```python
from build123d import *

# Parameters (mm, degrees)
SKETCH_1_R          = 135
EXTRUDE_1_DEPTH     = 2
SKETCH_562_R        = 1.6
SKETCH_562_W        = 21
SKETCH_562_H        = 44
CUT_EXTRUDE_1_DEPTH = 10
SKETCH_1031_R       = 1.6
CUT_EXTRUDE_2_DEPTH = 10
SKETCH_4_R          = 2
SKETCH_4_R_2        = 3
SKETCH_4_R_3        = 1.6
CUT_EXTRUDE_3_DEPTH = 10
CUT_EXTRUDE_4_DEPTH = 10
SKETCH_6_R          = 1.6
CUT_EXTRUDE_7_DEPTH = 10


with BuildPart() as part:
    # 草图1 → 凸台-拉伸1 (new body)
    with BuildSketch(Plane(origin=(0, 0, 0), x_dir=(1, 0, 0), z_dir=(0, 1, 0))):
        with Locations(Location((0, 0, 0), (0, 0, 270))):
            Circle(SKETCH_1_R)
    extrude(amount=EXTRUDE_1_DEPTH)

    # Sketch 562 → 切除-拉伸1 (cut)
    with BuildSketch(Plane(origin=(0, 2, 0), x_dir=(1, 0, 0), z_dir=(0, 1, 0))):
        with Locations(Location((-5, 64.75, 0), (0, 0, 270))):
            Circle(SKETCH_562_R)
        with Locations(Location((5, 64.75, 0), (0, 0, 270))):
            Circle(SKETCH_562_R)
        with Locations(Location((-5, 15.25, 0), (0, 0, 270))):
            Circle(SKETCH_562_R)
        with Locations(Location((5, 15.25, 0), (0, 0, 270))):
            Circle(SKETCH_562_R)
        with Locations(Location((18.5, 48.5, 0), (0, 0, 270))):
            Circle(SKETCH_562_R)
        with Locations(Location((18.5, 11.5, 0), (0, 0, 270))):
            Circle(SKETCH_562_R)
        with Locations(Location((-18.5, 11.5, 0), (0, 0, 270))):
            Circle(SKETCH_562_R)
        with Locations(Location((-18.5, 48.5, 0), (0, 0, 270))):
            Circle(SKETCH_562_R)
        with Locations((0, 40)):
            Rectangle(SKETCH_562_W, SKETCH_562_H)
    extrude(amount=-CUT_EXTRUDE_1_DEPTH, mode=Mode.SUBTRACT)

    # Sketch 1031 → 切除-拉伸2 (cut)
    with BuildSketch(Plane(origin=(0, 2, 0), x_dir=(1, 0, 0), z_dir=(0, 1, 0))):
        with Locations(Location((-60, -25, 0), (0, 0, 270))):
            Circle(SKETCH_1031_R)
        with Locations(Location((-40, -25, 0), (0, 0, 270))):
            Circle(SKETCH_1031_R)
        with Locations(Location((40, -25, 0), (0, 0, 270))):
            Circle(SKETCH_1031_R)
        with Locations(Location((60, -25, 0), (0, 0, 270))):
            Circle(SKETCH_1031_R)
        with Locations(Location((60, -105, 0), (0, 0, 270))):
            Circle(SKETCH_1031_R)
        with Locations(Location((40, -105, 0), (0, 0, 270))):
            Circle(SKETCH_1031_R)
        with Locations(Location((-40, -105, 0), (0, 0, 270))):
            Circle(SKETCH_1031_R)
        with Locations(Location((-60, -105, 0), (0, 0, 270))):
            Circle(SKETCH_1031_R)
        with Locations(Location((-42.5, -89.5, 0), (0, 0, 270))):
            Circle(SKETCH_1031_R)
        with Locations(Location((-42.5, -40.5, 0), (0, 0, 270))):
            Circle(SKETCH_1031_R)
        with Locations(Location((15.5, -40.5, 0), (0, 0, 270))):
            Circle(SKETCH_1031_R)
        with Locations(Location((15.5, -89.5, 0), (0, 0, 270))):
            Circle(SKETCH_1031_R)
    extrude(amount=-CUT_EXTRUDE_2_DEPTH, mode=Mode.SUBTRACT)

    # 草图4 → 切除-拉伸3 (cut)
    with BuildSketch(Plane(origin=(0, 2, 0), x_dir=(1, 0, 0), z_dir=(0, 1, 0))):
        with Locations(Location((-72, 97, 0), (0, 0, 270))):
            Circle(SKETCH_4_R)
        with Locations(Location((72, 97, 0), (0, 0, 270))):
            Circle(SKETCH_4_R)
        with Locations(Location((72, -97, 0), (0, 0, 270))):
            Circle(SKETCH_4_R)
        with Locations(Location((-72, -97, 0), (0, 0, 270))):
            Circle(SKETCH_4_R)
        with Locations(Location((0, -120, 0), (0, 0, 270))):
            Circle(SKETCH_4_R_2)
        with Locations(Location((-5.656854249, -125.656854249, 0), (0, 0, 270))):
            Circle(SKETCH_4_R_3)
        with Locations(Location((-5.656854249, -114.343145751, 0), (0, 0, 270))):
            Circle(SKETCH_4_R_3)
        with Locations(Location((5.656854249, -114.343145751, 0), (0, 0, 270))):
            Circle(SKETCH_4_R_3)
        with Locations(Location((5.656854249, -125.656854249, 0), (0, 0, 270))):
            Circle(SKETCH_4_R_3)
        with Locations(Location((5.656854249, 125.656854249, 0), (0, 0, 270))):
            Circle(SKETCH_4_R_3)
        with Locations(Location((5.656854249, 114.343145751, 0), (0, 0, 270))):
            Circle(SKETCH_4_R_3)
        with Locations(Location((-5.656854249, 114.343145751, 0), (0, 0, 270))):
            Circle(SKETCH_4_R_3)
        with Locations(Location((-5.656854249, 125.656854249, 0), (0, 0, 270))):
            Circle(SKETCH_4_R_3)
        with Locations(Location((0, 120, 0), (0, 0, 270))):
            Circle(SKETCH_4_R_2)
        with BuildLine():
            Line((-20, -12.5), (20, -12.5))
            ThreePointArc((20, -12.5), (27.5, -20), (20, -27.5))
            Line((20, -27.5), (-20, -27.5))
            ThreePointArc((-20, -27.5), (-27.5, -20), (-20, -12.5))
        make_face()
    extrude(amount=-CUT_EXTRUDE_3_DEPTH, mode=Mode.SUBTRACT)

    # 草图5 → 切除-拉伸4 (cut)
    with BuildSketch(Plane(origin=(0, 2, 0), x_dir=(1, 0, 0), z_dir=(0, 1, 0))):
        with BuildLine():
            Line((-31.36862915, 63.63137085), (-17.36862915, 49.63137085))
            ThreePointArc((-17.36862915, 49.63137085), (-17.36862915, 47.36862915), (-19.63137085, 47.36862915))
            Line((-19.63137085, 47.36862915), (-33.63137085, 61.36862915))
            ThreePointArc((-33.63137085, 61.36862915), (-33.63137085, 63.63137085), (-31.36862915, 63.63137085))
        make_face()
        with BuildLine():
            Line((33.63137085, 61.36862915), (19.63137085, 47.36862915))
            ThreePointArc((19.63137085, 47.36862915), (17.36862915, 47.36862915), (17.36862915, 49.63137085))
            Line((17.36862915, 49.63137085), (31.36862915, 63.63137085))
            ThreePointArc((31.36862915, 63.63137085), (33.63137085, 63.63137085), (33.63137085, 61.36862915))
        make_face()
        with BuildLine():
            Line((31.36862915, -3.63137085), (17.36862915, 10.36862915))
            ThreePointArc((17.36862915, 10.36862915), (17.36862915, 12.63137085), (19.63137085, 12.63137085))
            Line((19.63137085, 12.63137085), (33.63137085, -1.36862915))
            ThreePointArc((33.63137085, -1.36862915), (33.63137085, -3.63137085), (31.36862915, -3.63137085))
        make_face()
        with BuildLine():
            Line((-33.63137085, -1.36862915), (-19.63137085, 12.63137085))
            ThreePointArc((-19.63137085, 12.63137085), (-17.36862915, 12.63137085), (-17.36862915, 10.36862915))
            Line((-17.36862915, 10.36862915), (-31.36862915, -3.63137085))
            ThreePointArc((-31.36862915, -3.63137085), (-33.63137085, -3.63137085), (-33.63137085, -1.36862915))
        make_face()
    extrude(amount=-CUT_EXTRUDE_4_DEPTH, mode=Mode.SUBTRACT)

    # 草图6 → 切除-拉伸7 (cut)
    with BuildSketch(Plane(origin=(0, 2, 0), x_dir=(1, 0, 0), z_dir=(0, 1, 0))):
        with Locations(Location((71.537199543, 2.5, 0), (0, 0, 270))):
            Circle(SKETCH_6_R)
        with Locations(Location((90.537199543, 2.5, 0), (0, 0, 270))):
            Circle(SKETCH_6_R)
        with Locations(Location((90.537199543, 57.5, 0), (0, 0, 270))):
            Circle(SKETCH_6_R)
        with Locations(Location((71.537199543, 57.5, 0), (0, 0, 270))):
            Circle(SKETCH_6_R)
        with Locations(Location((-95.215957975, -4.25, 0), (0, 0, 270))):
            Circle(SKETCH_6_R)
        with Locations(Location((-56.715957975, -4.25, 0), (0, 0, 270))):
            Circle(SKETCH_6_R)
        with Locations(Location((-95.215957975, 64.25, 0), (0, 0, 270))):
            Circle(SKETCH_6_R)
        with Locations(Location((-56.715957975, 64.25, 0), (0, 0, 270))):
            Circle(SKETCH_6_R)
        with BuildLine():
            add(Edge.make_bspline(
                [(-58.031053316, 15), (-47.63874847, 15), (-52.834900893, 37.5), (-58.031053316, 60), (-63.227205738, 37.5), (-68.423358161, 15), (-58.031053316, 15)],
                knots=[0, 0, 0, 2.094395102, 2.094395102, 4.188790205, 4.188790205, 6.283185307, 6.283185307, 6.283185307], degree=2, weights=[1, 0.5, 1, 0.5, 1, 0.5, 1]))
        make_face()
        with BuildLine():
            add(Edge.make_bspline(
                [(58.031053316, 45), (47.63874847, 45), (52.834900893, 22.5), (58.031053316, 0), (63.227205738, 22.5), (68.423358161, 45), (58.031053316, 45)],
                knots=[0, 0, 0, 2.094395102, 2.094395102, 4.188790205, 4.188790205, 6.283185307, 6.283185307, 6.283185307], degree=2, weights=[1, 0.5, 1, 0.5, 1, 0.5, 1]))
        make_face()
    extrude(amount=-CUT_EXTRUDE_7_DEPTH, mode=Mode.SUBTRACT)


solid = part.part
```
Work out the finished part from the listing and answer in its coordinate system (mm). A direction names the side the tool comes from. Give positions to 0.01 mm unless a question says otherwise; leave off trailing zeros. Loops run counter-clockwise (first coordinate to the right, second up) from the corner with the lowest first, then second, coordinate; pieces in that order, holes last. Notation, with made-up numbers: (-16, -26) -> (35, -26) arc R21 cw to (35, 3) -> close; hole circle Ø2 at (-38, 19.25). An arc over 180 degrees is marked (long way). Put each result on its own line as item: value. Start each with the question number.
Item 1: This flat-tipped pin is pushed along its axis until it touches: P1, Ø1, axis at y = 1, z = -11, coming from the -X side. Where does it stop, or does it pass through?
Item 2: Which of the six approach directions +Z, -Z, +X, -X, +Y, -Y give full straight-line access (tool end or side, diameter ignored) to faces 1 (the face through (2, 0, -2)), 2 (the face through (24.27, 1.01, -56.53))?
Item 3: Find the intervals of material crossed by L1, parallel to X at y = 0.5, z = 25 (3 decimals); L2, parallel to Z at x = 91, y = 1.6; L3, parallel to X at y = 1.45, z = -57.5, in increasing order. Write a range as [from, to].
Item 4: The mould has two halves that part along X. Classify faces 3 (the face through (-119.77, 0.99, 62.29)), 4 (the face through (-24.47, 1.01, -56.73)), 5 (the face through (2, 2, -2)): released by +X, released by -X, zero draft, split by the parting line, or undercut.
Item 5: The part is cut by section A-A (x = -108). Give the vertices of the cut face in (y, z).
Item 6: The part is cut by section D-D (z = 73.5). Give the vertices of the cut face in (x, y).
Item 7: The part is cut by section B-B (y = 1.1). State how many separate pieces and enclosed holes the cut face has, then the cut area to 3 significant figures.
Answers below:
1. P1: x = -134.59
2. face 1: +Z, -Z, +X, -X, -Y
2. face 2: +Y, -Y
3. L1: [-132.665, -61.6], [-58.4, -41.6], [-38.4, -25.59], [25.59, 38.4], [41.6, 58.4], [61.6, 132.665]
3. L2: [-99.72, -59.03], [-55.97, -4.03], [-0.97, 99.72]
3. L3: [-122.14, -29.76], [-25.24, -10.5], [10.5, 25.24], [29.76, 69.94], [73.14, 88.94], [92.14, 122.14]
4. face 3: split by the parting line
4. face 4: undercut
4. face 5: zero draft
5. outline: (0, -81) -> (2, -81) -> (2, 81) -> (0, 81) -> close
6. outline: (-113.24, 0) -> (113.24, 0) -> (113.24, 2) -> (-113.24, 2) -> close
7. separate pieces: 1
7. enclosed holes: 46
7. area: 54,300 mm2
